The model under review builds one solid part; all positions refer to its coordinate system, in mm. Face numbers are marked on the shaded views. A direction names the side the tool comes from. Coordinates: 2 decimals unless noted, no trailing zeros. Loops run counter-clockwise (first coordinate to the right, second up) from the corner with the lowest first, then second, coordinate; pieces in that order, holes last. Notation, with made-up numbers: M -13.5,69 L 33.5,69 A27 cw 33.5,91 Z; hole C -9.5,88 d6. An arc over 180 degrees is marked long. Return JSON: item names as keys, results as strings.
```python
from build123d import *

# Parameters (mm, degrees)
F1_DEPTH = 250
F3_DEPTH = 80.001


with BuildPart() as f1:
    # F0 (on Front) → F1 (new body, symmetric)
    with BuildSketch(Plane.XZ):
        Polygon((-40, 0), (40, 0), (40, 120), (40, 200), (15, 200), (15, 120), (-15, 120), (-15, 200), (-40, 200), (-40, 120), align=None)
    extrude(amount=F1_DEPTH, both=True)

    # F2 (on face) → F3 (cut, through all)
    with BuildSketch(Plane.YZ.offset(40)):
        Polygon((-170, 72.962383), (-170, 0), (-50, 0), (-50, 90), (-170, 90), align=None)
        Polygon((50.587727, 0), (170.587727, 0), (170.587727, 72.962383), (170.587727, 90), (50.587727, 90), align=None)
    extrude(amount=-F3_DEPTH, mode=Mode.SUBTRACT)


solid = f1.part
```
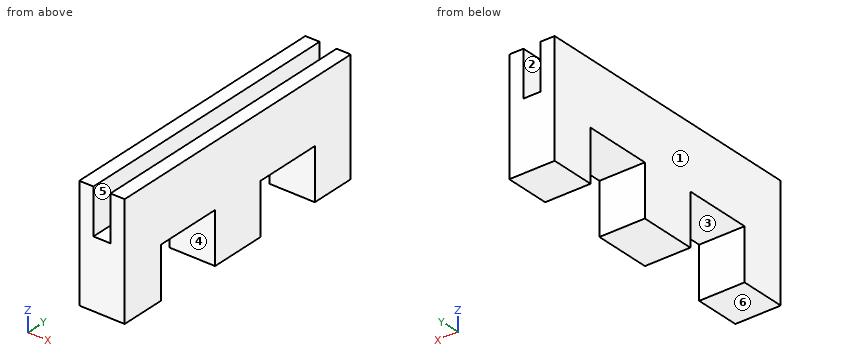
1. Add section B-B on y = -83.5. Give the boundary of the cut face in (x, z).
Check values:
{"outline": "M -40,90 L 40,90 L 40,200 L 15,200 L 15,120 L -15,120 L -15,200 L -40,200 Z"}
2. Add section D-D on x = -28. Give the boundary of the cut face in (y, z).
Check values:
{"outline": "M -250,0 L -170,0 L -170,90 L -50,90 L -50,0 L 50.59,0 L 50.59,90 L 170.59,90 L 170.59,0 L 250,0 L 250,200 L -250,200 Z"}
3. Insertion check: pin 1 Ø3 at (x, y) = (15.5, 144) entering from -Z. The pin has a flat end and moves straight along its axis. Give the tip position at first contact, or say it passes through.
Check values:
{"pin 1": "z = 90"}
4. Add section A-A on z = 150.5. Give the boundary of the cut face in (x, y).
Check values:
{"outline": "M -40,-250 L -15,-250 L -15,250 L -40,250 Z; M 15,-250 L 40,-250 L 40,250 L 15,250 Z"}
5. The part is to be moulded in two halves that separate along X. For the marked faces 1, 2 and 3, say which applies: released by +X, released by -X, zero draft, split by the parting line, or undercut.
Check values:
{"face 1": "released by -X", "face 2": "undercut", "face 3": "zero draft"}
6. Machinability: for the marked faces 4, 5 and 6, which of the approach directions +Z, -Z, +X, -X, +Y, -Y give a long, thin tool a straight path to every point of the face, cutting with its end or side? Answer none if there is none.
Check values:
{"face 4": "-Z, +X, -X", "face 5": "+Z, +Y, -Y", "face 6": "-Z, +X, -X, +Y, -Y"}
7. Add section C-C on z = 43. Give the boundary of the cut face in (x, y).
Check values:
{"outline": "M -40,-250 L 40,-250 L 40,-170 L -40,-170 Z; M -40,-50 L 40,-50 L 40,50.59 L -40,50.59 Z; M -40,170.59 L 40,170.59 L 40,250 L -40,250 Z"}
8. To check wall thickness, follow line 1 (Y direction, x = 31.5, z = 33.5); line 2 (X direction, y = -8, z = 124); line 3 (Z direction, x = -3.5, y = 130). State the ranges of each line that lie inside material, in increasing order.
Check values:
{"line 1": "-250 to -170, -50 to 50.59, 170.59 to 250", "line 2": "-40 to -15, 15 to 40", "line 3": "90 to 120"}
